For this review, take the finished solid that the model builds, in its own axes (mm). A direction names the side the tool comes from. Coordinates: 2 decimals unless noted, no trailing zeros. Write each loop counter-clockwise with the first axis right and the second up, starting at its lowest first coordinate (ties: lowest second). Pieces come first, ordered by that corner, then holes.
```python
from build123d import *

# Parameters (mm, degrees)
F0_W     = 5.800000261
F0_H     = 2.2
F0_W_2   = 2.2
F0_H_2   = 5.8
F1_DEPTH = 270
F2_R     = 5
F3_W     = 2.5
F3_H     = 20.3
F4_DEPTH = 25


with BuildPart() as f1:
    # F0 (on Right) → F1 (new body)
    with BuildSketch(Plane.YZ):
        Polygon((-14.3636103166, 75.9268823147), (-14.3636103166, 68.1268823147), (-14.3636103166, -0.2731176853), (-12.1636103166, -2.4731176853), (-12.1636103166, 68.1268823147), (-12.1636103166, 75.9268823147), align=None)
        Polygon((-12.1636103166, -2.4731176853), (-14.3636103166, -0.2731176853), (-14.3636103166, -3.3843875225), (-12.1636103166, -5.5843875225), align=None)
        with Locations((-17.2636104471, 77.0268823147)):
            Rectangle(F0_W, F0_H)
        with Locations((-13.2636103166, 77.0268823147)):
            Rectangle(F0_W_2, F0_H)
        Polygon((-7.7636103166, -6.8731176853), (-12.1636103166, -2.4731176853), (-12.1636103166, -5.5843875225), (-9.9636103166, -7.7843875225), (-9.9636103166, -35.9618478481), (-12.1636103166, -38.1618478481), (-12.1636103166, -41.2731176853), (-7.7636103166, -36.8731176853), align=None)
        Polygon((-14.3636103166, -43.4731176853), (-12.1636103166, -41.2731176853), (-12.1636103166, -38.1618478481), (-14.3636103166, -40.3618478481), align=None)
        Polygon((-12.1636103166, -92.4731176853), (-12.1636103166, -41.2731176853), (-14.3636103166, -43.4731176853), (-14.3636103166, -90.2731176853), align=None)
        Polygon((-7.7636103166, -96.8731176853), (-12.1636103166, -92.4731176853), (-12.1636103166, -95.5843875225), (-9.9636103166, -97.7843875225), (-9.9636103166, -125.9618478481), (-12.1636103166, -128.1618478481), (-12.1636103166, -131.2731176853), (-7.7636103166, -126.8731176853), align=None)
        Polygon((-12.1636103166, -95.5843875225), (-12.1636103166, -92.4731176853), (-14.3636103166, -90.2731176853), (-14.3636103166, -93.3843875225), align=None)
        Polygon((-14.3636103166, -133.4731176853), (-12.1636103166, -131.2731176853), (-12.1636103166, -128.1618478481), (-14.3636103166, -130.3618478481), align=None)
        Polygon((-12.1636103166, -179.6731176853), (-12.1636103166, -131.2731176853), (-14.3636103166, -133.4731176853), (-14.3636103166, -179.6731176853), align=None)
        Polygon((-12.1636103166, -181.8731176853), (-12.1636103166, -179.6731176853), (-14.3636103166, -179.6731176853), (-159.9636103166, -179.6731176853), (-159.9636103166, -181.8731176853), align=None)
        with Locations((-161.0636103166, -180.7731176853)):
            Rectangle(F0_W_2, F0_H)
        with Locations((-161.0636103166, -176.7731176853)):
            Rectangle(F0_W_2, F0_H_2)
    extrude(amount=F1_DEPTH)

    # F2
    f2_edges = [f1.edges().sort_by_distance(p)[0] for p in [
        (270, -161.06361, -173.873118),
        (0, -161.06361, -173.873118),
    ]]
    fillet(f2_edges, radius=F2_R)

    # F3 (on face) → F4 (cut)
    with BuildSketch(Plane.XY.offset(-179.6731176853)):
        with Locations((7.25, -134.8136103166)):
            Rectangle(F3_W, F3_H)
        with Locations((7.25, -102.8136103166)):
            Rectangle(F3_W, F3_H)
        with Locations((7.25, -70.8136103166)):
            Rectangle(F3_W, F3_H)
        with Locations((7.25, -38.8136103166)):
            Rectangle(F3_W, F3_H)
        with Locations((262.75, -134.8136103166)):
            Rectangle(F3_W, F3_H)
        with Locations((262.75, -102.8136103166)):
            Rectangle(F3_W, F3_H)
        with Locations((262.75, -70.8136103166)):
            Rectangle(F3_W, F3_H)
        with Locations((262.75, -38.8136103166)):
            Rectangle(F3_W, F3_H)
    extrude(amount=-F4_DEPTH, mode=Mode.SUBTRACT)


solid = f1.part
```
Q1. Draft analysis for pull direction Z (two halves, no side actions). For faces 1 (the flat face through (133, -12.164, -157)), 2 (the flat face through (133, -16, 78.127)), 3 (the flat face through (133, -88, -181.873)), 4 (the flat face through (133, -14.364, 37)), state which applies: +Z half, -Z half, draft (parallel to the pull), parting line (faces both ways), or undercut.
Ans:
face 1: draft
face 2: +Z half
face 3: -Z half
face 4: undercut
Q2. Add section B-B (x = 72). State the section outline as (y, z) points.
Ans:
outline: (-162.16, -181.87) - (-12.16, -181.87) - (-12.16, -131.27) - (-7.76, -126.87) - (-7.76, -96.87) - (-12.16, -92.47) - (-12.16, -41.27) - (-7.76, -36.87) - (-7.76, -6.87) - (-12.16, -2.47) - (-12.16, 78.13) - (-20.16, 78.13) - (-20.16, 75.93) - (-14.36, 75.93) - (-14.36, -3.38) - (-9.96, -7.78) - (-9.96, -35.96) - (-14.36, -40.36) - (-14.36, -93.38) - (-9.96, -97.78) - (-9.96, -125.96) - (-14.36, -130.36) - (-14.36, -179.67) - (-159.96, -179.67) - (-159.96, -173.87) - (-162.16, -173.87) - close
Q3. Tool access review of faces 5 (the flat face through (133, -12.164, -67)), 6 (the flat face through (133, -12.164, 37)), 7 (the flat face through (133, -9.964, -22)): name each direction out of +Z, -Z, +X, -X, +Y, -Y from which nothing blocks a thin tool from reaching the whole face with its end or side.
Ans:
face 5: +X, -X, +Y
face 6: +Z, +X, -X, +Y
face 7: +X, -X, -Y
Q4. For probe 1 along Z at (x, y) = (178, -14.5); probe 2 along Y at (x, z) = (192, 15); probe 3 along Z at (x, y) = (248.5, -38), list the stretches that pass through material, from the lowest coordinate up.
Ans:
probe 1: z = -181.87 to -179.67, 75.93 to 78.13
probe 2: y = -14.36 to -12.16
probe 3: z = -181.87 to -179.67
Q5. Add section A-A (y = -38.5). State the section outline as (x, z) points.
Ans:
outline: (0, -181.87) - (6, -181.87) - (6, -179.67) - (0, -179.67) - close; (8.5, -181.87) - (261.5, -181.87) - (261.5, -179.67) - (8.5, -179.67) - close; (264, -181.87) - (270, -181.87) - (270, -179.67) - (264, -179.67) - close
Q6. Add section C-C (z = 48). State the section outline as (x, y) points.
Ans:
outline: (0, -14.36) - (270, -14.36) - (270, -12.16) - (0, -12.16) - close
Q7. Clearance check with flat-ended pins moving along their axes: pin 1 Ø1.8 at (x, z) = (7, -180.5) entering from +Y; pin 2 Ø2 at (x, z) = (102.5, -27) entering from -Y; pin 3 Ø4 at (x, y) = (221.5, -110) entering from +Z. State where each tip first meets the part, or that it passes through.
Ans:
pin 1: stops at y = -12.16
pin 2: stops at y = -9.96
pin 3: stops at z = -179.67
